from build123d import *

# Parameters (mm, degrees)
SKETCH1_R           = 152.4
SKETCH1_R_2         = 139.7
BOSS_EXTRUDE1_DEPTH = 63.5
SKETCH2_W           = 34.925
SKETCH2_H           = 19.05
BOSS_EXTRUDE2_DEPTH = 38.1


with BuildPart() as part:
    # Sketch1 → Boss-Extrude1 (new, symmetric)
    with BuildSketch(Plane.XY):
        Circle(SKETCH1_R)
        Circle(SKETCH1_R_2, mode=Mode.SUBTRACT)
    extrude(amount=BOSS_EXTRUDE1_DEPTH, both=True)

    # Sketch2 → Boss-Extrude2 (add, symmetric)
    with BuildSketch(Plane.XY):
        with Locations((-131.7625, 0)):
            Rectangle(SKETCH2_W, SKETCH2_H)
    boss_extrude2 = extrude(amount=BOSS_EXTRUDE2_DEPTH, both=True)

    # Mirror2: Boss-Extrude2 across plane
    add(boss_extrude2.mirror(Plane(origin=(0, 0, 0), x_dir=(0, 0, 1), z_dir=(1, 0, 0))))


solid = part.part
Here's how the part is built. I have some questions about the finished solid (model axes, mm). A direction names the side the tool comes from. Round coordinates to 2 decimals unless told otherwise and drop trailing zeros. Loops run counter-clockwise (first coordinate to the right, second up) from the corner with the lowest first, then second, coordinate; pieces in that order, holes last. Notation, with made-up numbers: M -18.5,23.5 L 15.5,23.5 A10 cw 15.5,37.5 Z; hole C 18.25,23 d7. An arc over 180 degrees is marked long. Write each question's results on one line, items separated by ' | '. Start each with the question number.
(1) I want a section at B-B (y = 50). Please give me the cut outline in (x, z).
(2) I want a section at A-A (x = 0). Please give me the cut outline in (y, z).
(3) I want a section at C-C (z = 8.5). Please give me the cut outline in (x, y) (3 decimals), then the cut area to 3 significant figures.
(4) On a 3-axis mill with a long thin cutter (end or side, diameter ignored), from which of +Z, -Z, +X, -X, +Y, -Y can I reach the whole of each face in a straight line? I mean faces 1 (the flat face through (127, 0, 38.1)), 2 (the flat face through (67, -123, -63.5)), 3 (the flat face through (-127, 9.525, 1)), 4 (the flat face through (127, 0, -38.1)). Say none if no direction works.
(5) Will these pins go through, and if not, where does the flat tip stop? P1, Ø5.5, axis at x = 126.5, y = 3, coming from the -Z side; P2, Ø10, axis at y = 23.5, z = 50, coming from the -X side; P3, Ø4, axis at x = 90.5, z = -21.5, coming from the -Y side.
(6) If I drill on probe 1 along Y at (x, z) = (1, -43.5); probe 2 along Y at (x, z) = (-126, 21.5) (3 decimals); probe 3 along X at (y, z) = (-2, -26.5), over which ranges is the centre line in solid material (lowest first)? Write a range as from..to.
(7) I want a section at D-D (x = -124.5). Please give me the cut outline in (y, z) (3 decimals), then the cut area to 3 significant figures.
Solved:
1) outline: M -143.96,-63.5 L -130.45,-63.5 L -130.45,63.5 L -143.96,63.5 Z; M 130.45,-63.5 L 143.96,-63.5 L 143.96,63.5 L 130.45,63.5 Z
2) outline: M -152.4,-63.5 L -139.7,-63.5 L -139.7,63.5 L -152.4,63.5 Z; M 139.7,-63.5 L 152.4,-63.5 L 152.4,63.5 L 139.7,63.5 Z
3) outline: C 0,0 d304.8; hole M -139.375,-9.525 A139.7 ccw 139.375,-9.525 L 114.3,-9.525 L 114.3,9.525 L 139.375,9.525 A139.7 ccw -139.375,9.525 L -114.3,9.525 L -114.3,-9.525 Z | area: 12,600 mm²
4) face 1: +Z | face 2: -Z, +X, -X, +Y, -Y | face 3: +Z, -Z | face 4: -Z
5) P1: stops at z = -38.1 | P2: stops at x = -151.27 | P3: stops at y = -124.07
6) probe 1: y = -152.4..-139.7, 139.7..152.4 | probe 2: y = -85.731..-60.333, -9.525..9.525, 60.333..85.731 | probe 3: x = -152.39..-114.3, 114.3..152.39
7) outline: M -87.895,-63.5 L -63.371,-63.5 L -63.371,63.5 L -87.895,63.5 Z; M -9.525,-38.1 L 9.525,-38.1 L 9.525,38.1 L -9.525,38.1 Z; M 63.371,-63.5 L 87.895,-63.5 L 87.895,63.5 L 63.371,63.5 Z | area: 7,680 mm²
